Geometry check sheet. Reference: drawing and pictorial views, mm from the part's lowest x, y, z. Round coordinates to 2 decimals unless told otherwise and drop trailing zeros. Write each loop counter-clockwise with the first axis right and the second up, starting at its lowest first coordinate (ties: lowest second). Pieces come first, ordered by that corner, then holes. Notation, with made-up numbers: M -40,-8.5 L -9,-8.5 A36 ccw -9,25.5 Z; hole C 29.25,76 d9. An arc over 180 degrees is marked long. Answer in a Markdown table with one row per item. Add a question column.
1. Go/stop test with a flat-tipped pin: pin 1 Ø1.2 at (x, y) = (24.8, 6.8) entering from +Z. Record where the tip stops, or that it passes through.
2. Material ranges on probe 1 along Y at (x, z) = (24.8, 17.5); probe 2 along X at (y, z) = (7, 18.25), recorded low to high.
3. Sectioned sample at B-B on x = 3.2. Record the cut outline in (y, z).
4. Sectioned sample at A-A on y = 6.8. Record the cut outline in (x, z), plus the area to 3 significant figures.
5. Sectioned sample at C-C on z = 16. Record the cut outline in (x, y).
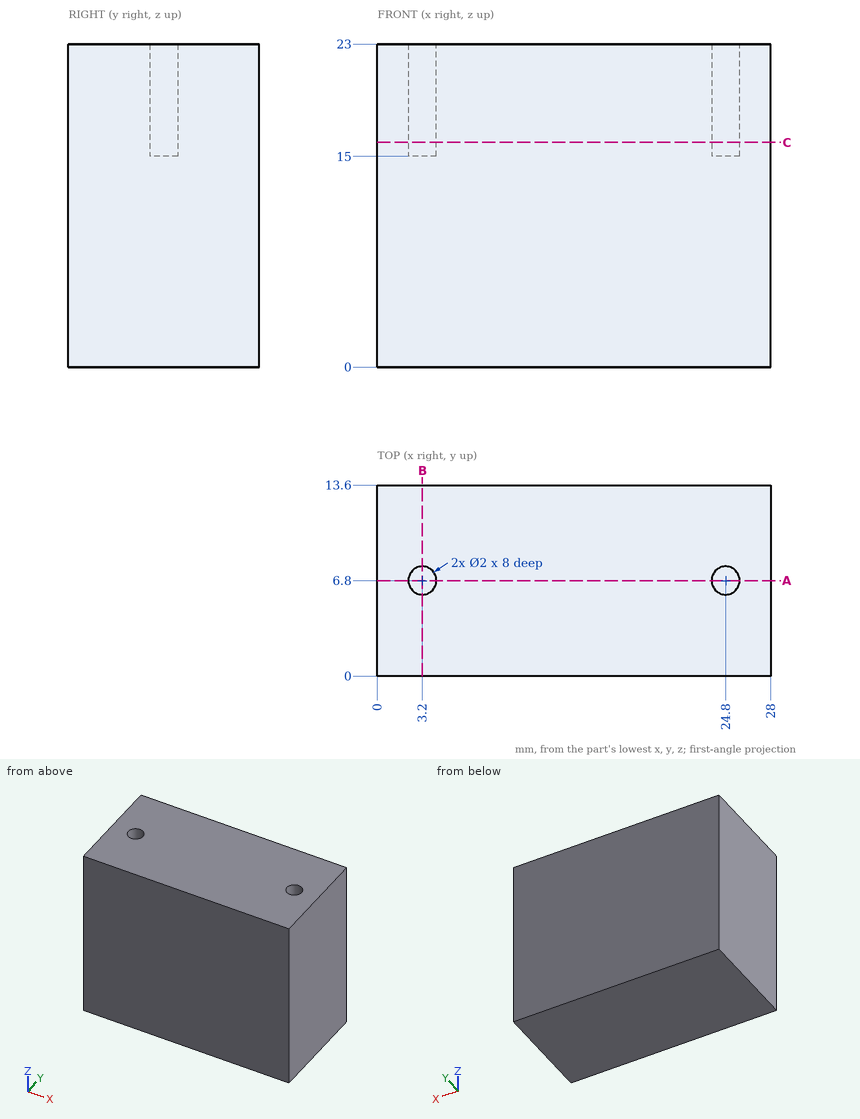
Geometry check:
| question | item | result |
|---|---|---|
| 1 | pin 1 | stops at z = 15 |
| 2 | probe 1 | y = 0 to 5.8, 7.8 to 13.6 |
| 2 | probe 2 | x = 0 to 2.22, 4.18 to 23.82, 25.78 to 28 |
| 3 | outline | M 0,0 L 13.6,0 L 13.6,23 L 7.8,23 L 7.8,15 L 5.8,15 L 5.8,23 L 0,23 Z |
| 4 | outline | M 0,0 L 28,0 L 28,23 L 25.8,23 L 25.8,15 L 23.8,15 L 23.8,23 L 4.2,23 L 4.2,15 L 2.2,15 L 2.2,23 L 0,23 Z |
| 4 | area | 612 mm2 |
| 5 | outline | M 0,0 L 28,0 L 28,13.6 L 0,13.6 Z; hole C 3.2,6.8 d2; hole C 24.8,6.8 d2 |
